Autodesk Inventor part; units mm, degrees
ref_plane "YZ Plane" through (0, 0, 0) normal (1, 0, 0) x (0, 1, 0)
ref_plane "XZ Plane" through (0, 0, 0) normal (0, 1, 0) x (-1, 0, 0)
ref_plane "XY Plane" through (0, 0, 0) normal (0, 0, 1) x (1, 0, 0)
sketch "Sketch1" plane through (0, 0, 0) normal (0, 0, 1) x (1, 0, 0)
  circle A0 centre (0, 6.35) radius 1.5875
  circle A1 centre (0, 0) radius 1.5875
  circle A2 centre (0, -6.35) radius 1.5875
  dimension "d0" = 3.175
  dimension "d1" = 6.35
  dimension "d2" = 6.35
extrude "Extrusion1" add sketch "Sketch1" along normal blind 6.35
sketch "Sketch2" plane through (0, 6.35, 6.35) normal (0, 0, 1) x (1, 0, 0)
  line L0 (-3.175, 3.175) -> (3.175, 3.175)
  line L1 (3.175, 3.175) -> (3.175, -15.875)
  line L2 (3.175, -15.875) -> (-3.175, -15.875)
  line L3 (-3.175, -15.875) -> (-3.175, 3.175)
  circle A0 centre (0, 0) radius 1.5875
  circle A1 centre (0, -12.7) radius 1.5875
  point P0 (0, -6.35)
  dimension "d5" = 6.35
  dimension "d7" = 3.175
  dimension "d8" = 3.175
  dimension "d11" = 3.175
extrude "Extrusion2" add sketch "Sketch2" along normal blind 6.35 contours L0 L1 L2 L3 | A0 | A1
sketch "Sketch3" plane through (-3.175, -9.525, 6.35) normal (0, -1, 0) x (1, 0, 0)
  line L0 (28.575, 25.4) -> (-22.225, 25.4)
  line L1 (-22.225, 25.4) -> (-22.225, -25.4)
  line L2 (-22.225, -25.4) -> (28.575, -25.4)
  line L3 (28.575, -25.4) -> (28.575, 25.4)
  line L4 (0, 0) -> (6.35, 0)
  line L5 (6.35, 0) -> (0, 0)
  line L6 (0, 0) -> (0, -13.97)
  line L7 (0, -13.97) -> (6.35, -13.97)
  line L8 (6.35, -13.97) -> (6.35, 0)
  point P0 (3.175, -6.35)
  dimension "d12" = 50.8
  dimension "d13" = 50.8
  dimension "d14" = 25.4
  dimension "d15" = 25.4
  dimension "d16" = 6.35
  dimension "d17" = 0
  dimension "d18" = 22.225
  dimension "d19" = 13.97
extrude "Extrusion3" add sketch "Sketch3" along normal blind 3.175
sketch "Sketch4" plane through (-3.175, -9.525, 6.35) normal (0, 1, 0) x (1, 0, 0)
  line L0 (-22.225, -25.4) -> (-22.225, 25.4)
  line L1 (-22.225, 25.4) -> (28.575, 25.4)
  line L2 (-22.225, -25.4) -> (28.575, -25.4)
  line L3 (28.575, -25.4) -> (28.575, 25.4)
  line L4 (28.575, 25.4) -> (-22.225, 25.4)
  line L5 (-22.225, 25.4) -> (-22.225, -25.4)
  line L6 (25.4, -22.225) -> (-19.05, -22.225)
  line L7 (-19.05, -22.225) -> (-19.05, 22.225)
  line L8 (-19.05, 22.225) -> (25.4, 22.225)
  line L9 (25.4, 22.225) -> (25.4, -22.225)
  point P0 (3.175, 6.35)
  dimension "d22" = 3.175
extrude "Extrusion4" add sketch "Sketch4" along normal blind 12.7
sketch "Sketch5" plane through (-3.175, -12.7, 6.35) normal (0, -1, 0) x (1, 0, 0)
  line L0 (6.35, 0) -> (6.35, -13.97)
  line L1 (0, -13.97) -> (0, 0)
  line L2 (6.35, 0) -> (0, 0)
  line L3 (0, 0) -> (0, -13.97)
  line L4 (0, -13.97) -> (6.35, -13.97)
  line L5 (6.35, -13.97) -> (6.35, 0)
  point P0 (3.175, -6.35)
extrude "Extrusion5" add sketch "Sketch5" against normal blind 1.5875
properties part number "Weight1"
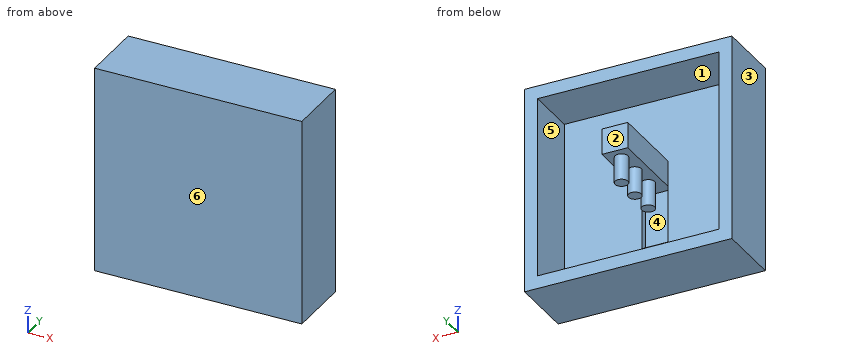
Source: CAD feature listing. Evaluate the final solid. Frame: model axes, mm. Face numbers are marked on the shaded views. A direction names the side the tool comes from. Coordinates: 2 decimals unless noted, no trailing zeros. Loops run counter-clockwise (first coordinate to the right, second up) from the corner with the lowest first, then second, coordinate; pieces in that order, holes last. Notation, with made-up numbers: (62, 52) - (114, 52) arc R19 cw to (114, 89) - close; hole circle Ø6 at (8, 65). An arc over 180 degrees is marked (long way). One line per question, with ' | ' between items.
1) Section A-A, the plane y = -2.25. Return loops of the section in (x, z) (3 decimals), then the cut area to 3 significant figures.
Report:
outline: (-25.4, -19.05) - (25.4, -19.05) - (25.4, 31.75) - (-25.4, 31.75) - close; (-3.175, 6.35) - (3.175, 6.35) - (3.175, 12.7) - (-3.175, 12.7) - close; hole (-22.225, -15.875) - (22.225, -15.875) - (22.225, 28.575) - (-22.225, 28.575) - close | area: 645 mm²
2) Set-up query: the marked faces 4, 5 and 6. Return all of +Z, -Z, +X, -X, +Y, -Y with unobstructed straight access to the full face (end or side cutting, diameter ignored); none if empty.
Report:
face 4: none | face 5: +Y | face 6: +Z, -Z, +X, -X, -Y
3) Line query: line 1 along Z through (x, y) = (2.5, -7.25) (3 decimals); line 2 along X through (y, z) = (-6.5, 5) (3 decimals); line 3 along Z through (x, y) = (-20, 1.75) (3 decimals). Output: solid intervals per line, ascending.
Report:
line 1: z = -19.05 to -15.875, 6.35 to 12.7, 28.575 to 31.75 | line 2: x = -25.4 to -22.225, -1.58 to 1.58, 22.225 to 25.4 | line 3: z = -19.05 to -15.875, 28.575 to 31.75
4) First-contact query: P1, Ø8, axis at x = 14.5, z = 23.5, coming from the +Y side (3 decimals); P2, Ø7, axis at x = 0.5, z = 0.5, coming from the +Y side; P3, Ø2.5, axis at x = -0.5, y = 6.5, coming from the -Z side. Flat tips, straight axial feed; report the tip coordinate or a pass-through.
Report:
P1: stops at y = -9.525 | P2: stops at y = 7.94 | P3: stops at z = 0
5) Section D-D, the plane z = 11. Return loops of the section in (x, y) (3 decimals), then the cut area to 3 significant figures.
Report:
outline: (-25.4, -12.7) - (25.4, -12.7) - (25.4, 3.175) - (22.225, 3.175) - (22.225, -9.525) - (3.175, -9.525) - (3.175, 9.525) - (-3.175, 9.525) - (-3.175, -9.525) - (-22.225, -9.525) - (-22.225, 3.175) - (-25.4, 3.175) - close | area: 363 mm²
6) Section C-C, the plane x = 5. Return loops of the section in (y, z) (3 decimals), then the cut area to 3 significant figures.
Report:
outline: (-12.7, -19.05) - (3.175, -19.05) - (3.175, -15.875) - (-9.525, -15.875) - (-9.525, 28.575) - (3.175, 28.575) - (3.175, 31.75) - (-12.7, 31.75) - close | area: 242 mm²
7) Section B-B, the plane z = 1.5. Give the number of separate pieces and of enclosed holes in the cut face, then the cut area to 3 significant figures.
Report:
separate pieces: 4 | enclosed holes: 0 | area: 256 mm²
8) Pull-direction query (X, two-part tool) for the marked faces 1, 2 and 3; classes: released by +X, released by -X, zero draft, split by the parting line, or undercut.
Report:
face 1: undercut | face 2: zero draft | face 3: released by -X
